Design review of the part built by this model. Coordinates are the model's own, in mm. A direction names the side the tool comes from. Give positions to 0.01 mm unless a question says otherwise; leave off trailing zeros. Write each loop counter-clockwise with the first axis right and the second up, starting at its lowest first coordinate (ties: lowest second). Pieces come first, ordered by that corner, then holes.
```python
from build123d import *

# Parameters (mm, degrees)
SKETCH_2_W               = 6
SKETCH_2_H               = 57
CUT_EXTRUDE_1_DEPTH      = 9
SKETCH_3_W               = 10
SKETCH_3_H               = 1.5
CUT_EXTRUDE_2_DEPTH      = 29.5
PATTERN_CIRCULAR_1_COUNT = 7


with BuildPart() as part:
    # Эскиз1 → Повернуть1 (revolve)
    with BuildSketch(Plane.XY):
        Polygon((24.5, 0), (24.5, 8), (28.5, 8), (28.5, 7), (27, 7), (27, 1), (28.5, 1), (28.5, 0), align=None)
    revolve(axis=Axis((0, 0, 0), (0, 1, 0)))

    # Эскиз2 → Вырез-Вытянуть1 (cut, through all)
    with BuildSketch(Plane(origin=(0, 0, 0), x_dir=(1, 0, 0), z_dir=(0, 1, 0))):
        with Locations((0, 28.5)):
            Rectangle(SKETCH_2_W, SKETCH_2_H)
    extrude(amount=CUT_EXTRUDE_1_DEPTH, mode=Mode.SUBTRACT)

    # Эскиз3 → Вырез-Вытянуть2 (cut, through all)
    with BuildSketch(Plane.XY):
        with Locations((0, 4)):
            Rectangle(SKETCH_3_W, SKETCH_3_H)
    cut_extrude_2 = extrude(amount=CUT_EXTRUDE_2_DEPTH, mode=Mode.SUBTRACT)

    # Круговой массив1: Вырез-Вытянуть2 ×7 about axis
    pattern_circular_1_axis = Axis((0, 0, 0), (0, 1, 0))
    for i in range(1, PATTERN_CIRCULAR_1_COUNT):
        add(cut_extrude_2.rotate(pattern_circular_1_axis, i * 360 / PATTERN_CIRCULAR_1_COUNT), mode=Mode.SUBTRACT)


solid = part.part
```
(1) Consider section B-B, the plane y = 4. Give the number of separate pieces and of enclosed holes in the cut face, then the cut area to 3 significant figures.
Resolved:
separate pieces: 8
enclosed holes: 0
area: 213 mm2
(2) Clearance check with flat-ended pins moving along their axes: P1, Ø2, axis at y = 2.5, z = -25.5, coming from the +X side; P2, Ø5.5, axis at x = 8.5, z = -21.5, coming from the -Y side; P3, Ø12, axis at x = -13, z = 9.5, coming from the -Y side; P4, Ø1.5, axis at y = 6.5, z = 18.5, coming from the -X side. State where each tip first meets the part, or that it passes through.
Resolved:
P1: stops at x = 11.35
P2: stops at y = 0
P3: passes through
P4: stops at x = -22.14
(3) Consider section C-C, the plane z = -22.5. Give the boundary of the cut face in (x, y), then the cut area to 3 significant figures.
Resolved:
outline: (-17.49, 0) - (-9.7, 0) - (-9.7, 3.25) - (-14.92, 3.25) - (-14.92, 1) - (-17.49, 1) - close; (-17.49, 7) - (-14.92, 7) - (-14.92, 4.75) - (-9.7, 4.75) - (-9.7, 8) - (-17.49, 8) - close; (9.7, 0) - (17.49, 0) - (17.49, 1) - (14.92, 1) - (14.92, 3.25) - (9.7, 3.25) - close; (9.7, 4.75) - (14.92, 4.75) - (14.92, 7) - (17.49, 7) - (17.49, 8) - (9.7, 8) - close
area: 78.3 mm2
(4) Consider section D-D, the plane x = -13. Give the boundary of the cut face in (y, z).
Resolved:
outline: (0, -25.36) - (1, -25.36) - (1, -23.66) - (3.25, -23.66) - (3.25, -20.77) - (0, -20.77) - close; (0, 20.77) - (8, 20.77) - (8, 25.36) - (7, 25.36) - (7, 23.66) - (1, 23.66) - (1, 25.36) - (0, 25.36) - close; (4.75, -23.66) - (7, -23.66) - (7, -25.36) - (8, -25.36) - (8, -20.77) - (4.75, -20.77) - close
(5) Tool access review of faces 3 (the face through (16.62, 3.99, 19.65)), 4 (the face through (5, 4, 25)), 5 (the face through (-3, 4, -26)), 6 (the face through (-15.456, 3.99, -20.572)), 7 (the face through (-1.211, 7.493, 28.474)): name each direction out of +Z, -Z, +X, -X, +Y, -Y from which nothing blocks a thin tool from reaching the whole face with its end or side.
Resolved:
face 3: +X
face 4: +Z
face 5: -Z, +Y, -Y
face 6: -Z
face 7: +Y, -Y
(6) Consider section A-A, the plane x = 0. Give the boundary of the cut face in (y, z).
Resolved:
outline: (0, 24.5) - (3.25, 24.5) - (3.25, 27) - (1, 27) - (1, 28.5) - (0, 28.5) - close; (4.75, 24.5) - (8, 24.5) - (8, 28.5) - (7, 28.5) - (7, 27) - (4.75, 27) - close
(7) Mouldability with a two-part tool opening along Y and no side actions: class faces 1 (the face through (0, 4.75, 25)), 2 (the face through (-1.211, 0.493, 28.474)) as pulls with the +Y half, pulls with the -Y half, needs draft (parallel to the pull), parting line crosses it, or undercut.
Resolved:
face 1: undercut
face 2: needs draft
(8) To check wall thickness, follow L1, parallel to X at y = 3.5, z = 0; L2, parallel to Y at x = -8.5, z = 26.5; L3, parallel to Z at x = 0, y = 6.25. State the ranges of each line that lie inside material, in increasing order.
Resolved:
L1: x = -27 to -24.5, 24.5 to 27
L2: y = 0 to 1, 7 to 8
L3: z = 24.5 to 27
